Can you work these out from the model? Positions are in its coordinate system, mm. A direction names the side the tool comes from. Round coordinates to 2 decimals unless told otherwise and drop trailing zeros. Loops run counter-clockwise (first coordinate to the right, second up) from the corner with the lowest first, then second, coordinate; pieces in that order, holes last. Notation, with made-up numbers: M -4.75,-29.5 L 10.25,-29.5 A11 ccw 10.25,-12.5 Z; hole C 75,55 d7. An arc over 180 degrees is marked long. Use a Markdown table: item, result. Add a question column.
```python
from build123d import *

# Parameters (mm, degrees)
ESQUISSE1_W             = 12
ESQUISSE1_H             = 15
BOSS_EXTRU_1_DEPTH      = 5
ESQUISSE2_W             = 10
ESQUISSE2_H             = 5
ESQUISSE2_H_2           = 3
BOSS_EXTRU_2_DEPTH      = 5
ESQUISSE3_R             = 1.5
ENL_V_MAT_EXTRU_1_DEPTH = 5
ESQUISSE4_R             = 3
ENL_V_MAT_EXTRU_2_DEPTH = 10


with BuildPart() as part:
    # Esquisse1 → Boss.-Extru.1 (new body)
    with BuildSketch(Plane(origin=(0, 0, 0), x_dir=(1, 0, 0), z_dir=(0, 1, 0))):
        with Locations((1, 0)):
            Rectangle(ESQUISSE1_W, ESQUISSE1_H)
    extrude(amount=BOSS_EXTRU_1_DEPTH)

    # Esquisse2 → Boss.-Extru.2 (add)
    with BuildSketch(Plane(origin=(0, 5, 0), x_dir=(1, 0, 0), z_dir=(0, 1, 0))):
        with Locations((0, 10)):
            Rectangle(ESQUISSE2_W, ESQUISSE2_H)
        with Locations((0, -9)):
            Rectangle(ESQUISSE2_W, ESQUISSE2_H_2)
    extrude(amount=-BOSS_EXTRU_2_DEPTH)

    # Esquisse3 → Enlèv. mat.-Extru.1 (cut)
    with BuildSketch(Plane(origin=(0, 5, 0), x_dir=(1, 0, 0), z_dir=(0, 1, 0))):
        with Locations((1, 10)):
            Circle(ESQUISSE3_R)
    extrude(amount=-ENL_V_MAT_EXTRU_1_DEPTH, mode=Mode.SUBTRACT)

    # Esquisse4 → Enlèv. mat.-Extru.2 (cut)
    with BuildSketch(Plane(origin=(0, 5, 0), x_dir=(1, 0, 0), z_dir=(0, 1, 0))):
        Circle(ESQUISSE4_R)
    extrude(amount=-ENL_V_MAT_EXTRU_2_DEPTH, mode=Mode.SUBTRACT)


solid = part.part
```
(1) Suppose I cut it at D-D on z = -9.5. List the corners of the cut face in (x, y) for me, and give its area (3 significant figures).
(2) Thinking about a two-plate mould opening in Z: for faces 1 (the face through (0, 3, -12.5)), 2 (the face through (-5, 3, -1)), 3 (the face through (0.675, 2.535, -8.536)), 4 (the face through (6, 2, 7.5)), which applies, released by +Z, released by -Z, zero draft, split by the parting line, or undercut?
(3) Suppose I cut it at B-B on y = 2.35. List the corners of the cut face in (x, z) for me, and give its area (3 significant figures).
(4) On a 3-axis mill with a long thin cutter (end or side, diameter ignored), from which of +Z, -Z, +X, -X, +Y, -Y can I reach the whole of each face in a straight line? I mean faces 5 (the face through (5, 3, 9)), 6 (the face through (6, 2, -7.5)), 7 (the face through (-3, 3, 0)). Say none if no direction works.
(5) Suppose I cut it at A-A on z = 0. List the corners of the cut face in (x, y) for me.
(6) I'm going to push flat-ended pins straight in: pin 1 (5 mm diameter, centred on x = 1, z = -10, fed in from +Y); pin 2 (2.5 mm diameter, centred on y = 2, z = -9, fed in from +X); pin 3 (0.6 mm diameter, centred on x = 6.5, y = 2, fed in from -Z). Where does each tip first touch, or does it pass through?
(7) Suppose I cut it at C-C on x = 1. List the corners of the cut face in (y, z) for me.
(8) If I drill on probe 1 along X at (y, z) = (1.1, -10); probe 2 along X at (y, z) = (1.6, 0); probe 3 along Z at (x, y) = (0, 3.1), over which ranges is the centre line in solid material (lowest first)? Write a range as [from, to].
Results below:
| question | item | result |
|---|---|---|
| 1 | outline | M -5,0 L -0.41,0 L -0.41,5 L -5,5 Z; M 2.41,0 L 5,0 L 5,5 L 2.41,5 Z |
| 1 | area | 35.9 mm² |
| 2 | face 1 | released by -Z |
| 2 | face 2 | zero draft |
| 2 | face 3 | undercut |
| 2 | face 4 | released by +Z |
| 3 | outline | M -5,-12.5 L 5,-12.5 L 5,-7.5 L 7,-7.5 L 7,7.5 L 5,7.5 L 5,10.5 L -5,10.5 Z; hole C 0,0 d6; hole C 1,-10 d3 |
| 3 | area | 225 mm² |
| 4 | face 5 | +Z, +X, +Y, -Y |
| 4 | face 6 | -Z, +X, +Y, -Y |
| 4 | face 7 | +Y, -Y |
| 5 | outline | M -5,0 L -3,0 L -3,5 L -5,5 Z; M 3,0 L 7,0 L 7,5 L 3,5 Z |
| 6 | pin 1 | stops at y = 5 |
| 6 | pin 2 | stops at x = 5 |
| 6 | pin 3 | stops at z = -7.5 |
| 7 | outline | M 0,-12.5 L 5,-12.5 L 5,-11.5 L 0,-11.5 Z; M 0,-8.5 L 5,-8.5 L 5,-2.83 L 0,-2.83 Z; M 0,2.83 L 5,2.83 L 5,10.5 L 0,10.5 Z |
| 8 | probe 1 | x = [-5, -0.5], [2.5, 5] |
| 8 | probe 2 | x = [-5, -3], [3, 7] |
| 8 | probe 3 | z = [-12.5, -11.12], [-8.88, -3], [3, 10.5] |
